Input: part model. Units: mm. Frame: model coordinates. A direction names the side the tool comes from. Round coordinates to 2 decimals unless told otherwise and drop trailing zeros. Loops run counter-clockwise (first coordinate to the right, second up) from the corner with the lowest first, then second, coordinate; pieces in that order, holes last. Notation, with made-up numbers: M 23,27 L 49,27 A15 cw 49,54 Z; hole C 74,22.25 d11. An arc over 180 degrees is marked long. Put each result on its own line as item: value. Start each with the question number.
1) Reachability of faces 3 (the face through (0, 0, 0)), 4 (the face through (-2, 2, -7)), 5 (the face through (-2, 2, -228)) from +Z, -Z, +X, -X, +Y, -Y: full face, straight path, thin tool, end or side. Return the list, or none.
2) Section A-A on y = 0. Output: boundary loops of the cut face in (x, z).
3) Section C-C on z = -122. Output: boundary loops of the cut face in (x, y), plus the area to 3 significant figures.
4) Draft query along Y for faces 1 (the face through (0, 0, -235)), 2 (the face through (-3.233, -1.341, -119.047)). Return one class per face: +Y half, -Y half, draft (parallel to the pull), parting line (faces both ways), or undercut.
5) Line query: probe 1 along Z at (x, y) = (3, 1); probe 2 along X at (y, z) = (-0.5, -209); probe 3 along Y at (x, z) = (-0.25, -85.5). Output: solid intervals per line, ascending.
6) Pin query (flat end, axial travel): pin 1 (1.5 mm diameter, centred on x = 3, z = -31, fed in from -Y). Return the tip coordinate at first contact, or that it passes through.
Autodesk Inventor part; units mm, degrees
ref_plane "YZ Plane" through (0, 0, 0) normal (1, 0, 0) x (0, 1, 0)
ref_plane "XZ Plane" through (0, 0, 0) normal (0, 1, 0) x (-1, 0, 0)
ref_plane "XY Plane" through (0, 0, 0) normal (0, 0, 1) x (1, 0, 0)
sketch "Skizze1" plane through (0, 0, 0) normal (0, 1, 0) x (-1, 0, 0)
  line L0 (0, 0) -> (2.5, 0)
  line L1 (2.5, 0) -> (2.5, -7)
  line L2 (2.5, -7) -> (3.5, -7)
  line L3 (3.5, -7) -> (3.5, -228)
  line L4 (3.5, -228) -> (2.5, -228)
  line L5 (2.5, -228) -> (2.5, -235)
  line L6 (2.5, -235) -> (0, -235)
  line L7 (0, -235) -> (0, 0)
  dimension "d0" = 7
  dimension "d1" = 5
  dimension "d2" = 7
  dimension "d3" = 7
  dimension "d4" = 235
revolve "Umdrehung1" add sketch "Skizze1" angle 360 about axis through (0, 0, -235) along (0, 0, 1)
equation "\"d3\" = d2"
properties part number "2071"
Geometry results:
1. face 3: +Z, +X, -X, +Y, -Y
1. face 4: +Z
1. face 5: -Z
2. outline: M -3.5,-228 L -2.5,-228 L -2.5,-235 L 2.5,-235 L 2.5,-228 L 3.5,-228 L 3.5,-7 L 2.5,-7 L 2.5,0 L -2.5,0 L -2.5,-7 L -3.5,-7 Z
3. outline: C 0,0 d7
3. area: 38.5 mm²
4. face 1: draft
4. face 2: parting line
5. probe 1: z = -228 to -7
5. probe 2: x = -3.46 to 3.46
5. probe 3: y = -3.49 to 3.49
6. pin 1: stops at y = -2.68
